from build123d import *

# Parameters (mm, degrees)
F0_R          = 10.375
F0_R_2        = 8.875
F1_DEPTH      = 2
F1_DEPTH_BACK = 2
F2_SIZE       = 1
F4_START      = 9.775
F3_R          = 0.7
F4_DEPTH      = 15.225
F5_R          = 0.5
F6_DEPTH      = 9.3


with BuildPart() as f1:
    # F0 (on Front) → F1 (new body, two sides)
    with BuildSketch(Plane.XZ) as f1_sk:
        Circle(F0_R)
        Circle(F0_R_2, mode=Mode.SUBTRACT)
    extrude(amount=F1_DEPTH)
    extrude(f1_sk.sketch, amount=-F1_DEPTH_BACK)

    # F2
    f2_edges = [f1.edges().sort_by_distance(p)[0] for p in [
        (-8.875, -2, 0),
        (-8.875, 2, 0),
    ]]
    chamfer(f2_edges, length=F2_SIZE)

    # F3 (on Top) → F4 (cut)
    with BuildSketch(Plane.XY.offset(F4_START)):
        with BuildLine():
            Line((-1.5, -1), (1.5, -1))
            ThreePointArc((1.5, -1), (2.2071067812, -0.7071067812), (2.5, 0))
            ThreePointArc((2.5, 0), (2.2071067812, 0.7071067812), (1.5, 1))
            Line((1.5, 1), (-1.5, 1))
            ThreePointArc((-1.5, 1), (-2.2071067812, 0.7071067812), (-2.5, 0))
            ThreePointArc((-2.5, 0), (-2.2071067812, -0.7071067812), (-1.5, -1))
        make_face()
        Circle(F3_R, mode=Mode.SUBTRACT)
    extrude(amount=F4_DEPTH, mode=Mode.SUBTRACT)

    # F5 (on Top) → F6 (cut)
    with BuildSketch(Plane.XY):
        with BuildLine():
            ThreePointArc((1.7263360261, -2.2374776466), (1.521310773, -1.7425028998), (1.0263360261, -1.5374776466))
            Line((1.0263360261, -1.5374776466), (-1.0660886515, -1.5374776466))
            ThreePointArc((-1.0660886515, -1.5374776466), (-1.5610633983, -1.7425028998), (-1.7660886515, -2.2374776466))
            ThreePointArc((-1.7660886515, -2.2374776466), (-1.5610633983, -2.7324523935), (-1.0660886515, -2.9374776466))
            Line((-1.0660886515, -2.9374776466), (1.0263360261, -2.9374776466))
            ThreePointArc((1.0263360261, -2.9374776466), (1.521310773, -2.7324523935), (1.7263360261, -2.2374776466))
        make_face()
        with BuildLine():
            ThreePointArc((1.7563359968, -0.0024776423), (1.5513107436, 0.4924971045), (1.0563359968, 0.6975223577))
            Line((1.0563359968, 0.6975223577), (-1.0360886808, 0.6975223577))
            ThreePointArc((-1.0360886808, 0.6975223577), (-1.5310634277, 0.4924971045), (-1.7360886808, -0.0024776423))
            ThreePointArc((-1.7360886808, -0.0024776423), (-1.5310634277, -0.4974523892), (-1.0360886808, -0.7024776423))
            Line((-1.0360886808, -0.7024776423), (1.0563359968, -0.7024776423))
            ThreePointArc((1.0563359968, -0.7024776423), (1.5513107436, -0.4974523892), (1.7563359968, -0.0024776423))
        make_face()
        with Locations((0.0053813122, -0.0004659606)):
            Circle(F5_R, mode=Mode.SUBTRACT)
        with BuildLine():
            ThreePointArc((1.7263360261, 2.2689716425), (1.521310773, 2.7639463893), (1.0263360261, 2.9689716425))
            Line((1.0263360261, 2.9689716425), (-1.0660886515, 2.9689716425))
            ThreePointArc((-1.0660886515, 2.9689716425), (-1.5610633983, 2.7639463893), (-1.7660886515, 2.2689716425))
            ThreePointArc((-1.7660886515, 2.2689716425), (-1.5610633983, 1.7739968956), (-1.0660886515, 1.5689716425))
            Line((-1.0660886515, 1.5689716425), (1.0263360261, 1.5689716425))
            ThreePointArc((1.0263360261, 1.5689716425), (1.521310773, 1.7739968956), (1.7263360261, 2.2689716425))
        make_face()
    extrude(amount=-F6_DEPTH, mode=Mode.SUBTRACT)


solid = f1.part
Source: CAD feature listing. Evaluate the final solid. Frame: model axes, mm. A direction names the side the tool comes from. Give positions to 0.01 mm unless a question says otherwise; leave off trailing zeros. Write each loop counter-clockwise with the first axis right and the second up, starting at its lowest first coordinate (ties: lowest second). Pieces come first, ordered by that corner, then holes. Notation, with made-up numbers: (27, -27) - (77, -27) arc R22 cw to (77, 1) - close; hole circle Ø3 at (25.25, -6.75). An arc over 180 degrees is marked (long way). Write item = value, one per line. Start each with the question number.
Q1. Cut plane C-C, the plane y = -0.25. Return loops of the section in (x, z) (3 decimals), then the cut area to 3 significant figures.
Q2. Cut plane D-D, the plane y = 1.3. Return loops of the section in (x, z) (3 decimals), then the cut area to 3 significant figures.
Q3. Reachability of faces 1 (the cylindrical face through (0.47, -0.19, -9.08)), 2 (the cylindrical face through (-2.25, -0.03, -10.13)), 3 (the cylindrical face through (-0.7, 0, 10.1)) from +Z, -Z, +X, -X, +Y, -Y: full face, straight path, thin tool, end or side. Return the list, or none.
Q4. Cut plane A-A, the plane z = 0. Return loops of the section in (x, y) (3 decimals), then the cut area to 4 significant figures.
Q5. Material intervals for probe 1 along Z at (x, y) = (0, 0.65) (3 decimals); probe 2 along Z at (x, y) = (0, 0.3) (3 decimals); probe 3 along X at (y, z) = (0.2, -7.75), sorted ascending.
Q6. Draft query along X for faces 4 (the cylindrical face through (-0.002, 0.007, -8.875)), 5 (the cylindrical face through (0.01, -0.01, 10.375)), 6 (the flat face through (-1, 0, 9.775)). Return one class per face: +X half, -X half, draft (parallel to the pull), parting line (faces both ways), or undercut.
Q7. Pin query (flat end, axial travel): pin 1 Ø4 at (x, z) = (6.5, -4) entering from +Y; pin 2 Ø0.5 at (x, z) = (0, -9) entering from +Y (3 decimals); pin 3 Ø1 at (x, z) = (-7.5, -1) entering from -Y. Return the tip coordinate at first contact, or that it passes through.
Computed values:
q1.outline = (-2.468, 9.775) - (-2.468, 10.077) arc R10.375 ccw (long way) to (2.468, 10.077) - (2.468, 9.775) - (0.654, 9.775) - (0.654, 10.354) arc R10.375 ccw to (-0.654, 10.354) - (-0.654, 9.775) - close; hole (-1.691, -9.3) - (-0.428, -9.3) - (-0.428, -8.865) arc R8.875 ccw to (0.439, -8.864) - (0.439, -9.3) - (1.711, -9.3) - (1.711, -8.708) arc R8.875 ccw (long way) to (-1.691, -8.712) - close
q1.area = 87.8 mm²
q2.outline = circle Ø20.75 at (0, 0); hole circle Ø18.35 at (0, 0)
q2.area = 73.7 mm²
q3.face_1 = none
q3.face_2 = +Y, -Y
q3.face_3 = +Z
q4.outline = (-10.375, -2) - (-9.875, -2) - (-8.875, -1) - (-8.875, 1) - (-9.875, 2) - (-10.375, 2) - close; (8.875, -1) - (9.875, -2) - (10.375, -2) - (10.375, 2) - (9.875, 2) - (8.875, 1) - close
q4.area = 10.00 mm²
q5.probe_1 = -10.375 to -9.3, 8.875 to 10.375
q5.probe_2 = -10.375 to -8.875, 8.875 to 10.375
q5.probe_3 = -6.9 to -4.32, 4.32 to 6.9
q6.face_4 = undercut
q6.face_5 = parting line
q6.face_6 = undercut
q7.pin_1 = 1.76
q7.pin_2 = 1.375
q7.pin_3 = through
